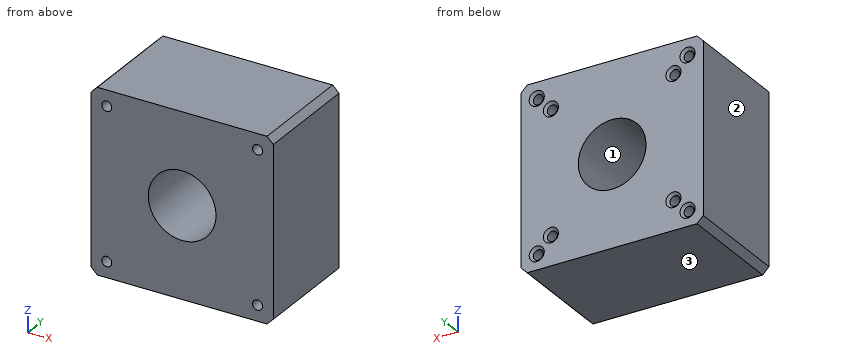
```python
from build123d import *

# Parameters (mm, degrees)
SKETCH1_W                        = 73.66
SKETCH1_H                        = 73.66
SKETCH1_R                        = 13.6921875
BOSS_EXTRUDE1_DEPTH              = 43.65625
CHAMFER2_SIZE                    = 2.54
F_10_32_TAPPED_HOLE1_D           = 4.0386
F_10_32_TAPPED_HOLE1_CSINK_D     = 6.096
F_10_32_TAPPED_HOLE1_CSINK_ANGLE = 90
F_10_32_TAPPED_HOLE2_D           = 4.0386
F_10_32_TAPPED_HOLE2_DEPTH       = 21.844
F_10_32_TAPPED_HOLE2_CSINK_D     = 6.096
F_10_32_TAPPED_HOLE2_CSINK_ANGLE = 90
F_10_32_TAPPED_HOLE2_TIP         = 1.213317848


with BuildPart() as part:
    # Sketch1 → Boss-Extrude1 (new body)
    with BuildSketch(Plane(origin=(0, 0, 0), x_dir=(1, 0, 0), z_dir=(0, 1, 0))):
        Rectangle(SKETCH1_W, SKETCH1_H)
        with Locations(Location((0, 0, 0), (0, 0, 270))):
            Circle(SKETCH1_R, mode=Mode.SUBTRACT)
    extrude(amount=BOSS_EXTRUDE1_DEPTH)

    # Chamfer2
    chamfer2_edges = [part.edges().sort_by_distance(p)[0] for p in [
        (-36.83, 21.828125, -36.83),
        (36.83, 21.828125, -36.83),
        (36.83, 21.828125, 36.83),
        (-36.83, 21.828125, 36.83),
    ]]
    chamfer(chamfer2_edges, length=CHAMFER2_SIZE)

    # #10-32 Tapped Hole1 (through all)
    with Locations(Plane(origin=(0, 43.65625, 0), x_dir=(1, 0, 0), z_dir=(0, 1, 0))):
        with Locations((30.48, 30.48), (-30.48, 30.48), (-30.48, -30.48), (30.48, -30.48)):
            CounterSinkHole(F_10_32_TAPPED_HOLE1_D / 2, F_10_32_TAPPED_HOLE1_CSINK_D / 2, counter_sink_angle=F_10_32_TAPPED_HOLE1_CSINK_ANGLE)

    # #10-32 Tapped Hole2
    with Locations(Plane(origin=(0, 43.65625, 0), x_dir=(1, 0, 0), z_dir=(0, 1, 0))):
        with Locations((-24.765, 24.765), (24.765, 24.765), (-24.765, -24.765), (24.765, -24.765)):
            CounterSinkHole(F_10_32_TAPPED_HOLE2_D / 2, F_10_32_TAPPED_HOLE2_CSINK_D / 2, depth=F_10_32_TAPPED_HOLE2_DEPTH, counter_sink_angle=F_10_32_TAPPED_HOLE2_CSINK_ANGLE)
            with Locations((0, 0, -(F_10_32_TAPPED_HOLE2_DEPTH + F_10_32_TAPPED_HOLE2_TIP / 2))):  # 118° drill point
                Cone(0, F_10_32_TAPPED_HOLE2_D / 2, F_10_32_TAPPED_HOLE2_TIP, mode=Mode.SUBTRACT)


solid = part.part
```
Input: part model. Units: mm. Frame: model coordinates. Face numbers are marked on the shaded views. Coordinates: 2 decimals unless noted, no trailing zeros. Order: outer loops, then holes, each group sorted by start corner. A loop starts at its lowest first (then second) coordinate and runs counter-clockwise, first axis right, second up. Notation, with made-up numbers: (13.5, -34.75) - (56.5, -34.75) arc R21 ccw to (56.5, -1.75) - close; hole circle Ø3 at (-31, 12.25). An arc over 180 degrees is marked (long way). Return JSON: item names as keys, results as strings.
Q1. Cut plane B-B (y = 11). Return loops of the section in (x, z), then the cut area to 3 significant figures.
The answers:
{"outline": "(-36.83, -34.29) - (-34.29, -36.83) - (34.29, -36.83) - (36.83, -34.29) - (36.83, 34.29) - (34.29, 36.83) - (-34.29, 36.83) - (-36.83, 34.29) - close; hole circle Ø4.04 at (-30.48, -30.48); hole circle Ø4.04 at (-30.48, 30.48); hole circle Ø27.38 at (0, 0); hole circle Ø4.04 at (30.48, -30.48); hole circle Ø4.04 at (30.48, 30.48)", "area": "4,770 mm2"}
Q2. Cut plane A-A (z = 30.48). Return loops of the section in (x, y), then the cut area to 3 significant figures.
The answers:
{"outline": "(-36.83, 0) - (-32.5, 0) - (-32.5, 42.63) - (-33.53, 43.66) - (-36.83, 43.66) - close; (-28.46, 0) - (28.46, 0) - (28.46, 42.63) - (27.43, 43.66) - (-27.43, 43.66) - (-28.46, 42.63) - close; (32.5, 0) - (36.83, 0) - (36.83, 43.66) - (33.53, 43.66) - (32.5, 42.63) - close", "area": "2,860 mm2"}
Q3. Cut plane D-D (y = 34). State how many separate pieces and enclosed holes the cut face has, then the cut area to 3 significant figures.
The answers:
{"separate pieces": "1", "enclosed holes": "9", "area": "4,720 mm2"}
Q4. Ray query, probe 1 along X at (y, z) = (31.5, 30.48); probe 2 along X at (y, z) = (34, -30). Return the intervals inside material, ascending.
The answers:
{"probe 1": "x = -36.83 to -32.5, -28.46 to 28.46, 32.5 to 36.83", "probe 2": "x = -36.83 to -32.44, -28.52 to 28.52, 32.44 to 36.83"}
Q5. Draft query along Z for the marked faces 1, 2 and 3. Return one class per face: +Z half, -Z half, draft (parallel to the pull), parting line (faces both ways), or undercut.
The answers:
{"face 1": "undercut", "face 2": "draft", "face 3": "-Z half"}
Q6. Cut plane C-C (x = -30.48). Return loops of the section in (y, z), then the cut area to 3 significant figures.
The answers:
{"outline": "(0, -36.83) - (43.66, -36.83) - (43.66, -33.53) - (42.63, -32.5) - (0, -32.5) - close; (0, -28.46) - (42.63, -28.46) - (43.66, -27.43) - (43.66, 27.43) - (42.63, 28.46) - (0, 28.46) - close; (0, 32.5) - (42.63, 32.5) - (43.66, 33.53) - (43.66, 36.83) - (0, 36.83) - close", "area": "2,860 mm2"}
Q7. First-contact query: pin 1 (3 mm diameter, centred on x = -24.765, z = -24.765, fed in from +Y); pin 2 (5.5 mm diameter, centred on x = -30.48, z = -30.48, fed in from +Y); pin 3 (2.5 mm diameter, centred on x = 30.48, z = 30.48, fed in from -Y); pin 4 (4.5 mm diameter, centred on x = 24.765, z = -24.765, fed in from +Y). Flat tips, straight axial feed; report the tip coordinate or a pass-through.
The answers:
{"pin 1": "stops at y = 21.5", "pin 2": "stops at y = 43.36", "pin 3": "passes through", "pin 4": "stops at y = 42.86"}
